from build123d import *

# Parameters (mm, degrees)
ESBO_O1_R                     = 40
ESBO_O1_R_2                   = 30
RESSALTO_EXTRUS_O1_DEPTH      = 50
ESBO_O2_R                     = 1.5
CORTE_EXTRUS_O1_DEPTH         = 6
CORTE_EXTRUS_O2_DEPTH         = 11.84997677
RESSALTO_EXTRUS_O2_DEPTH      = 26.84997677
RESSALTO_EXTRUS_O2_DEPTH_BACK = 10


with BuildPart() as part:
    # Esboço1 → Ressalto-extrusão1 (new body)
    with BuildSketch(Plane(origin=(0, 0, 0), x_dir=(1, 0, 0), z_dir=(0, 1, 0))):
        with Locations(Location((0, 0, 0), (0, 0, 270))):
            Circle(ESBO_O1_R)
        with Locations(Location((0, 0, 0), (0, 0, 270))):
            Circle(ESBO_O1_R_2, mode=Mode.SUBTRACT)
    extrude(amount=RESSALTO_EXTRUS_O1_DEPTH)

    # Esboço2 → Corte-extrusão1 (cut)
    with BuildSketch(Plane(origin=(0, 0, 0), x_dir=(-1, 0, 0), z_dir=(0, -1, 0))):
        with Locations(Location((-21.160269083, -29.124611797, 0), (0, 0, 90))):
            Circle(ESBO_O2_R)
        with Locations(Location((-34.238034587, -11.124611797, 0), (0, 0, 90))):
            Circle(ESBO_O2_R)
        with Locations(Location((-34.238034587, 11.124611797, 0), (0, 0, 90))):
            Circle(ESBO_O2_R)
        with Locations(Location((21.160269083, 29.124611797, 0), (0, 0, 90))):
            Circle(ESBO_O2_R)
        with Locations(Location((34.238034587, 11.124611797, 0), (0, 0, 90))):
            Circle(ESBO_O2_R)
        with Locations(Location((34.238034587, -11.124611797, 0), (0, 0, 90))):
            Circle(ESBO_O2_R)
    extrude(amount=-CORTE_EXTRUS_O1_DEPTH, mode=Mode.SUBTRACT)

    # Esboço3 → Corte-extrusão2 (cut)
    with BuildSketch(Plane(origin=(0, 0, 0), x_dir=(-1, 0, 0), z_dir=(0, -1, 0))):
        with BuildLine():
            ThreePointArc((30.293924668, -13.087327008), (31.253408489, 10.593604572), (16.092357529, 28.81034587))
            Line((16.092357529, 28.81034587), (19.505887914, 34.921631358))
            ThreePointArc((19.505887914, 34.921631358), (8.030354378, 39.185627576), (-4.197370073, 39.779166463))
            Line((-4.197370073, 39.779166463), (-3.148027555, 29.834374847))
            ThreePointArc((-3.148027555, 29.834374847), (29.911212101, 2.306380417), (1.462902849, -29.964310692))
            Line((1.462902849, -29.964310692), (1.950537132, -39.952414256))
            ThreePointArc((1.950537132, -39.952414256), (22.185986252, -33.283359416), (36.126859334, -17.171197823))
            Line((36.126859334, -17.171197823), (30.293924668, -13.087327008))
        make_face()
    extrude(amount=-CORTE_EXTRUS_O2_DEPTH, mode=Mode.SUBTRACT)

    # Esboço4 → Ressalto-extrusão2 (add, two sides: drawn at the far end of the back side and taken through both)
    with BuildSketch(Plane(origin=(0, 11.84997677, 0), x_dir=(-1, 0, 0), z_dir=(0, -1, 0)).offset(-RESSALTO_EXTRUS_O2_DEPTH_BACK)):
        with BuildLine():
            Line((-4.008838629, -29.730947056), (-4.700362463, -27.602655537))
            ThreePointArc((-4.700362463, -27.602655537), (-8.119302432, 26.79695744), (19.230258499, -20.351834268))
            Line((19.230258499, -20.351834268), (19.909240802, -22.441526924))
            ThreePointArc((19.909240802, -22.441526924), (-8.745833796, 28.696870757), (-4.008838629, -29.730947056))
        make_face()
    extrude(amount=RESSALTO_EXTRUS_O2_DEPTH + RESSALTO_EXTRUS_O2_DEPTH_BACK)


solid = part.part
Input: part model. Units: mm. Frame: model coordinates. A direction names the side the tool comes from. Coordinates: 2 decimals unless noted, no trailing zeros. Order: outer loops, then holes, each group sorted by start corner. A loop starts at its lowest first (then second) coordinate and runs counter-clockwise, first axis right, second up. Notation, with made-up numbers: M -30,39.25 L 27,39.25 A20 cw 27,78.25 Z; hole C 83.25,57.25 d4. An arc over 180 degrees is marked long. Answer as CSV lines item,"result".
1. First-contact query: P1, Ø10, axis at x = -1, y = -7, coming from the -Z side; P2, Ø1, axis at y = 26.5, z = 24.5, coming from the -X side; P3, Ø2.5, axis at x = -20.5, z = -28.5, coming from the -Y side. Flat tips, straight axial feed; report the tip coordinate or a pass-through.
Reported:
P1,"z = -30"
P2,"x = -32"
P3,"y = 0"
2. Section C-C (x = 1.5). Return the cut outline in (y, z).
Reported:
outline,"M -15,-29.96 L 11.85,-29.96 L 11.85,-39.97 L 50,-39.97 L 50,-29.96 L 21.85,-29.96 L 21.85,-27.96 L -15,-27.96 Z; M 0,29.96 L 50,29.96 L 50,39.97 L 0,39.97 Z"
3. Section B-B (y = 2). Return the cut outline in (x, z).
Reported:
outline,"M -36.13,17.17 A40 ccw -19.51,-34.92 L -16.09,-28.81 A33 cw -30.29,13.09 Z; M -19.91,22.44 A30 ccw 3.15,-29.83 L 4.2,-39.78 A40 ccw -1.95,39.95 L -1.46,29.96 A30 cw 4.01,29.73 L 4.7,27.6 A28 cw long -19.23,20.35 Z; hole C -34.24,-11.12 d3; hole C -34.24,11.12 d3; hole C -21.16,-29.12 d3; hole C 21.16,29.12 d3; hole C 34.24,-11.12 d3; hole C 34.24,11.12 d3"
4. Section A-A (z = 0). Return the cut outline in (x, y).
Reported:
outline,"M -40,0 L -33,0 L -33,11.85 L -30,11.85 L -30,-15 L -28,-15 L -28,21.85 L -30,21.85 L -30,50 L -40,50 Z; M 28,-15 L 30,-15 L 30,0 L 40,0 L 40,50 L 30,50 L 30,21.85 L 28,21.85 Z"
5. Access query for faces 1 (the cylindrical face through (32.9, 3, -11.8)), 2 (the flat face through (-33.251, 5.842, 15.158)), 3 (the flat face through (13, 21.85, -25)), 4 (the flat face through (-32, 0, -11)), 5 (the flat face through (-1.703, 5.842, 34.888)). Directions: +Z, -Z, +X, -X, +Y, -Y. A direction counts if a zero-diameter tool reaches every point of the face in a straight line with its end or side. Return the directions, or none.
Reported:
face 1,"-Y"
face 2,"+Z, -Y"
face 3,"+Y"
face 4,"-Z, -X, -Y"
face 5,"-X, -Y"
6. Pull-direction query (Z, two-part tool) for faces 6 (the flat face through (-17.775, 5.842, -31.823)), 7 (the flat face through (13, -15, -25)), 8 (the flat face through (4.35, 3.68, 28.68)); classes: released by +Z, released by -Z, zero draft, split by the parting line, or undercut.
Reported:
face 6,"released by -Z"
face 7,"zero draft"
face 8,"undercut"
7. Material intervals for line 1 (X direction, y = 3, z = 0); line 2 (Z direction, x = 0, y = 17); line 3 (X direction, y = 8.5, z = -25.5), sorted ascending. Write a range as from..to.
Reported:
line 1,"-40..-33, -30..-28, 28..40"
line 2,"-40..-28, 30..40"
line 3,"-30.82..-20.95, -15.8..-11.57, 11.57..30.82"
8. Section D-D (y = 19). Return the cut outline in (x, z).
Reported:
outline,"C 0,0 d80; hole M -19.91,22.44 L -19.23,20.35 A28 ccw long 4.7,27.6 L 4.01,29.73 A30 ccw Z"
